For this review, take the finished solid that the model builds, in its own axes (mm). Give positions to 0.01 mm unless a question says otherwise; leave off trailing zeros. Order: outer loops, then holes, each group sorted by start corner. A loop starts at its lowest first (then second) coordinate and runs counter-clockwise, first axis right, second up. Notation, with made-up numbers: (73, 35) - (121, 35) arc R22 cw to (121, 73) - close; hole circle Ø11 at (7.25, 25.5). An arc over 180 degrees is marked (long way). Use a Markdown table: item, result. Add a question column.
1) We need section B-B on y = -8. Write out the cut boundary in (x, z), then the cut area to 3 significant figures.
2) We need section D-D on y = 7. Write out the cut boundary in (x, z).
3) Wall thickness on L1, parallel to Y at x = 0, z = 4.5 (3 decimals); L2, parallel to X at y = 27.94, z = 1.5 (3 decimals); L3, parallel to Y at x = 1, z = 1.25: over which ranges is each line inside the solid? List them lowest first.
4) Mouldability with a two-part tool opening along Y and no side actions: class faces 1 (the face through (14, 3, 0)), 2 (the face through (0.176, -20.956, 3.219)), 3 (the face through (0.978, 30.298, 3.219)) as released by +Y, released by -Y, zero draft, split by the parting line, or undercut.
5) We need section A-A on x = 0. Write out the cut boundary in (y, z) (3 decimals).
6) We need section C-C on z = 0.75. Write out the cut boundary in (x, y) (1 decimal), then the cut area to 3 significant figures.
7) Clearance check with flat-ended pins moving along their axes: P1, Ø3, axis at y = 23, z = 1.5, coming from the -X side; P2, Ø1, axis at y = 24.5, z = 4, coming from the +X side. State where each tip first meets the part, or that it passes through.
Autodesk Inventor part; units mm, degrees
ref_plane "YZ Plane" through (0, 0, 0) normal (1, 0, 0) x (0, 1, 0)
ref_plane "XZ Plane" through (0, 0, 0) normal (0, 1, 0) x (-1, 0, 0)
ref_plane "XY Plane" through (0, 0, 0) normal (0, 0, 1) x (1, 0, 0)
sketch "Sketch1" plane through (0, 0, 0) normal (0, 0, 1) x (1, 0, 0)
  circle A0 centre (0, 0) radius 13.97
  circle A1 centre (0, 0) radius 34.925
  circle A2 centre (0, 0) radius 27.94
  point P0 (0, 27.94)
  point P1 (-26.5725, 8.6339)
  point P2 (-16.4227, -22.6039)
  point P3 (16.4227, -22.6039)
  point P4 (26.5725, 8.6339)
  dimension "d2" = 55.88
  dimension "d0" = 27.94
  dimension "d1" = 69.85
  dimension "d5" = 360
extrude "Extrusion1" add sketch "Sketch1" along normal blind 6.35 contours A1 | A2
hole "Hole1" at (0, 27.94, 0) at (-26.5725, 8.6339, 0) at (-16.4227, -22.6039, 0) at (16.4227, -22.6039, 0) at (26.5725, 8.6339, 0) direction (0, 0, 1) diameter 5.1054 end through all
thread "Thread1"
thread "Thread2"
thread "Thread3"
thread "Thread4"
thread "Thread5"
sketch "Sketch2" plane through (0, 0, 6.35) normal (0, 0, 1) x (1, 0, 0)
  circle A0 centre (0, 27.94) radius 2.5527
  circle A1 centre (-26.5725, 8.6339) radius 2.5527
  circle A2 centre (-16.4227, -22.6039) radius 2.5527
  circle A3 centre (16.4227, -22.6039) radius 2.5527
  circle A4 centre (26.5725, 8.6339) radius 2.5527
  circle A5 centre (-26.5725, 8.6339) radius 6.985
  circle A6 centre (0, 27.94) radius 6.985
  circle A7 centre (26.5725, 8.6339) radius 6.985
  circle A8 centre (16.4227, -22.6039) radius 6.985
  circle A9 centre (-16.4227, -22.6039) radius 6.985
  circle A10 centre (0, 0) radius 34.925
  circle A11 centre (0, 0) radius 20.955
  arc A12 (-24.2449, 15.2197) -> (-6.9827, 27.7615) centre (-19.9294, 27.4305) ccw
  arc A13 (-21.9669, -18.3552) -> (-28.5605, 1.9378) centre (-32.2464, -10.4775) ccw
  arc A14 (10.6686, -26.5638) -> (-10.6686, -26.5638) centre (0, -33.9059) ccw
  arc A15 (28.5605, 1.9378) -> (21.9669, -18.3552) centre (32.2464, -10.4775) ccw
  arc A16 (6.9827, 27.7615) -> (24.2449, 15.2197) centre (19.9294, 27.4305) ccw
  point P0 (-28.5605, 1.9378)
  point P1 (-33.2156, 10.7924)
  point P2 (-20.5284, -28.2549)
  point P3 (-21.9669, -18.3552)
  point P4 (0, 34.925)
  point P5 (33.2156, 10.7924)
  point P6 (6.9827, 27.7615)
  point P7 (21.9669, -18.3552)
  point P8 (20.5284, -28.2549)
  point P9 (28.5605, 1.9378)
  point P10 (-10.6686, -26.5638)
  point P11 (10.6686, -26.5638)
  dimension "d29" = 360
extrude "Extrusion2" cut sketch "Sketch2" against normal blind 25.4 contours A5 A10 A6 A12 | A5 A13 A9 A10 | A10 A7 A16 A6 | A9 A14 A8 A10 | A10 A8 A15 A7
properties part number "panel_flange"
Checked values:
| question | item | result |
|---|---|---|
| 1 | outline | (-19.53, 0) - (-11.45, 0) - (-11.45, 6.35) - (-19.53, 6.35) - close; (11.45, 0) - (19.53, 0) - (19.53, 6.35) - (11.45, 6.35) - close |
| 1 | area | 103 mm² |
| 2 | outline | (-33.36, 0) - (-28.53, 0) - (-28.53, 6.35) - (-33.36, 6.35) - close; (-24.61, 0) - (-12.09, 0) - (-12.09, 6.35) - (-24.61, 6.35) - close; (12.09, 0) - (24.61, 0) - (24.61, 6.35) - (12.09, 6.35) - close; (28.53, 0) - (33.36, 0) - (33.36, 6.35) - (28.53, 6.35) - close |
| 3 | L1 | -20.955 to -13.97, 13.97 to 25.387, 30.493 to 34.925 |
| 3 | L2 | -6.985 to -2.553, 2.553 to 6.985 |
| 3 | L3 | -20.99 to -13.93, 13.93 to 25.59, 30.29 to 34.85 |
| 4 | face 1 | zero draft |
| 4 | face 2 | released by -Y |
| 4 | face 3 | undercut |
| 5 | outline | (-20.955, 0) - (-13.97, 0) - (-13.97, 6.35) - (-20.955, 6.35) - close; (13.97, 0) - (25.387, 0) - (25.387, 6.35) - (13.97, 6.35) - close; (30.493, 0) - (34.925, 0) - (34.925, 6.35) - (30.493, 6.35) - close |
| 6 | outline | (-28.6, 1.9) arc R13 cw to (-22, -18.4) arc R7 ccw (long way) to (-10.7, -26.6) arc R13 cw to (10.7, -26.6) arc R7 ccw (long way) to (22, -18.4) arc R13 cw to (28.6, 1.9) arc R7 ccw (long way) to (24.2, 15.2) arc R13 cw to (7, 27.8) arc R7 ccw (long way) to (-7, 27.8) arc R13 cw to (-24.2, 15.2) arc R7 ccw (long way) to start; hole circle Ø5.1 at (-26.6, 8.6); hole circle Ø5.1 at (-16.4, -22.6); hole circle Ø27.9 at (0, 0); hole circle Ø5.1 at (0, 27.9); hole circle Ø5.1 at (16.4, -22.6); hole circle Ø5.1 at (26.6, 8.6) |
| 6 | area | 1,650 mm² |
| 7 | P1 | x = -8.42 |
| 7 | P2 | x = 7.44 |
